from build123d import *

# Parameters (mm, degrees)
SKETCH_1_R          = 5
EXTRUDE_1_DEPTH     = 10
SKETCH_2_R          = 7.5
CUT_EXTRUDE_1_DEPTH = 153.397506541


with BuildPart() as part:
    # 草图1 → 凸台-拉伸1 (new body)
    with BuildSketch(Plane.XY):
        with BuildLine():
            Line((-95, -110), (95, -110))
            ThreePointArc((95, -110), (102.071067812, -107.071067812), (105, -100))
            Line((105, -100), (105, 100))
            ThreePointArc((105, 100), (102.071067812, 107.071067812), (95, 110))
            Line((95, 110), (-95, 110))
            ThreePointArc((-95, 110), (-102.071067812, 107.071067812), (-105, 100))
            Line((-105, 100), (-105, -100))
            ThreePointArc((-105, -100), (-102.071067812, -107.071067812), (-95, -110))
        make_face()
        with Locations((97.5, 0)):
            Circle(SKETCH_1_R, mode=Mode.SUBTRACT)
        with Locations((0, 102.5)):
            Circle(SKETCH_1_R, mode=Mode.SUBTRACT)
        with Locations((60, 102.5)):
            Circle(SKETCH_1_R, mode=Mode.SUBTRACT)
        with Locations((97.5, 50)):
            Circle(SKETCH_1_R, mode=Mode.SUBTRACT)
        with Locations(Location((97.5, -50, 0), (0, 0, 180))):
            Circle(SKETCH_1_R, mode=Mode.SUBTRACT)
        with Locations(Location((60, -102.5, 0), (0, 0, 180))):
            Circle(SKETCH_1_R, mode=Mode.SUBTRACT)
        with Locations(Location((0, -102.5, 0), (0, 0, 180))):
            Circle(SKETCH_1_R, mode=Mode.SUBTRACT)
        with Locations(Location((-60, 102.5, 0), (0, 0, 180))):
            Circle(SKETCH_1_R, mode=Mode.SUBTRACT)
        with Locations((-60, -102.5)):
            Circle(SKETCH_1_R, mode=Mode.SUBTRACT)
        with Locations((-97.5, -50)):
            Circle(SKETCH_1_R, mode=Mode.SUBTRACT)
        with Locations(Location((-97.5, 0, 0), (0, 0, 180))):
            Circle(SKETCH_1_R, mode=Mode.SUBTRACT)
        with Locations(Location((-97.5, 50, 0), (0, 0, 180))):
            Circle(SKETCH_1_R, mode=Mode.SUBTRACT)
    extrude(amount=EXTRUDE_1_DEPTH)

    # 草图2 → 切除-拉伸1 (cut, through all)
    with BuildSketch(Plane.XY.offset(10)):
        Circle(SKETCH_2_R)
    extrude(amount=-CUT_EXTRUDE_1_DEPTH, mode=Mode.SUBTRACT)


solid = part.part
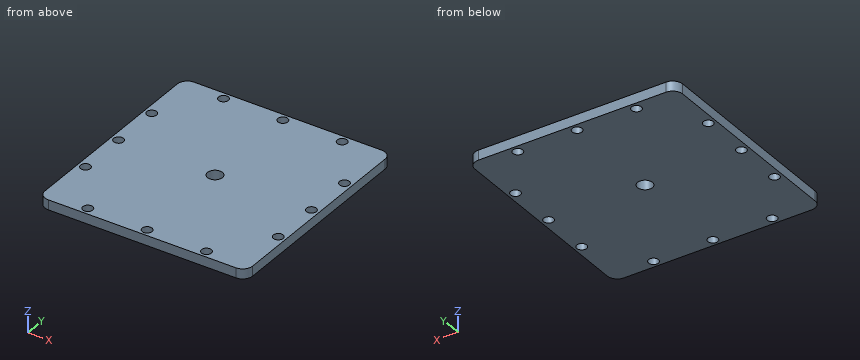
Geometry: final body of the model. Coordinates: model frame, mm. Give positions to 0.01 mm unless a question says otherwise; leave off trailing zeros. Order: outer loops, then holes, each group sorted by start corner. A loop starts at its lowest first (then second) coordinate and runs counter-clockwise, first axis right, second up. Notation, with made-up numbers: (-22, -24.75) -> (-3, -24.75) arc R23 ccw to (-3, -16.75) -> close; hole circle Ø9 at (-10.75, -14). An arc over 180 degrees is marked (long way). Answer as a JSON object with one key per item and string values.
Q1. Section D-D (x = -60). Output: boundary loops of the cut face in (y, z).
Entries:
{"outline": "(-110, 0) -> (-107.5, 0) -> (-107.5, 10) -> (-110, 10) -> close; (-97.5, 0) -> (97.5, 0) -> (97.5, 10) -> (-97.5, 10) -> close; (107.5, 0) -> (110, 0) -> (110, 10) -> (107.5, 10) -> close"}
Q2. Section C-C (z = 3.25). State how many separate pieces and enclosed holes the cut face has, plus the area to 3 significant figures.
Entries:
{"separate pieces": "1", "enclosed holes": "13", "area": "45,000 mm^2"}
Q3. Material intervals for probe 1 along X at (y, z) = (-49.5, 6); probe 2 along X at (y, z) = (-53, 2.5); probe 3 along Y at (x, z) = (-60, 7.25), sorted ascending.
Entries:
{"probe 1": "x = -105 to -102.47, -92.53 to 92.53, 102.47 to 105", "probe 2": "x = -105 to -101.5, -93.5 to 93.5, 101.5 to 105", "probe 3": "y = -110 to -107.5, -97.5 to 97.5, 107.5 to 110"}
Q4. Section A-A (x = 0). Output: boundary loops of the cut face in (y, z).
Entries:
{"outline": "(-110, 0) -> (-107.5, 0) -> (-107.5, 10) -> (-110, 10) -> close; (-97.5, 0) -> (-7.5, 0) -> (-7.5, 10) -> (-97.5, 10) -> close; (7.5, 0) -> (97.5, 0) -> (97.5, 10) -> (7.5, 10) -> close; (107.5, 0) -> (110, 0) -> (110, 10) -> (107.5, 10) -> close"}
Q5. Section B-B (y = -50). Output: boundary loops of the cut face in (x, z), plus the area to 3 significant figures.
Entries:
{"outline": "(-105, 0) -> (-102.5, 0) -> (-102.5, 10) -> (-105, 10) -> close; (-92.5, 0) -> (92.5, 0) -> (92.5, 10) -> (-92.5, 10) -> close; (102.5, 0) -> (105, 0) -> (105, 10) -> (102.5, 10) -> close", "area": "1,900 mm^2"}
Q6. First-contact query: pin 1 (8 mm diameter, centred on x = 97.5, y = -50, fed in from -Z). Flat tip, straight axial feed; report the tip coordinate or a pass-through.
Entries:
{"pin 1": "passes through"}
